For this review, take the finished solid that the model builds, in its own axes (mm). Round coordinates to 2 decimals unless told otherwise and drop trailing zeros. Write each loop counter-clockwise with the first axis right and the second up, starting at its lowest first coordinate (ties: lowest second). Pieces come first, ordered by that corner, then holes. Notation, with made-up numbers: (53.25, 35.5) -> (63.25, 35.5) arc R16 cw to (63.25, 52.5) -> close; hole circle Ø2 at (89, 30). An arc over 180 degrees is marked (long way). Answer in a Markdown table with one row per item.
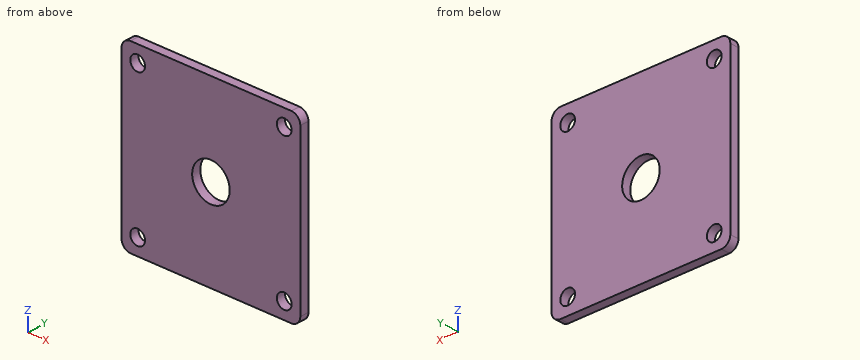
from build123d import *

# Parameters (mm, degrees)
SKETCH1_W           = 63.5
SKETCH1_H           = 63.5
BOSS_EXTRUDE1_DEPTH = 3.175
FILLET1_R           = 3.175
CUT_EXTRUDE1_REACH  = 47.013
SKETCH2_R           = 6.6675
CUT_EXTRUDE2_REACH  = 47.013
SKETCH3_R           = 2.6162


with BuildPart() as part:
    # Sketch1 → Boss-Extrude1 (new body)
    with BuildSketch(Plane(origin=(0, 0, 0), x_dir=(1, 0, 0), z_dir=(0, 1, 0))):
        Rectangle(SKETCH1_W, SKETCH1_H)
    extrude(amount=BOSS_EXTRUDE1_DEPTH)

    # Fillet1
    fillet1_edges = [part.edges().sort_by_distance(p)[0] for p in [
        (31.75, 1.5875, 31.75),
        (-31.75, 1.5875, 31.75),
        (-31.75, 1.5875, -31.75),
        (31.75, 1.5875, -31.75),
    ]]
    fillet(fillet1_edges, radius=FILLET1_R)

    # Sketch2 → Cut-Extrude1 (cut, up to next)
    with BuildSketch(Plane(origin=(0, 3.175, 0), x_dir=(1, 0, 0), z_dir=(0, 1, 0)), mode=Mode.PRIVATE) as cut_extrude1_sk1:
        with Locations(Location((0, 0, 0), (0, 0, 270))):
            Circle(SKETCH2_R)
    cut_extrude1_tool1 = extrude(cut_extrude1_sk1.sketch, amount=-CUT_EXTRUDE1_REACH, mode=Mode.PRIVATE) & part.part
    add(cut_extrude1_tool1.solids().sort_by_distance((0, 3.175, 0))[0], mode=Mode.SUBTRACT)

    # Sketch3 → Cut-Extrude2 (cut, up to next)
    with BuildSketch(Plane(origin=(0, 3.175, 0), x_dir=(1, 0, 0), z_dir=(0, 1, 0)), mode=Mode.PRIVATE) as cut_extrude2_sk1:
        with Locations(Location((26.042742751, -26.042742751, 0), (0, 0, 270))):
            Circle(SKETCH3_R)
    cut_extrude2_tool1 = extrude(cut_extrude2_sk1.sketch, amount=-CUT_EXTRUDE2_REACH, mode=Mode.PRIVATE) & part.part
    # Sketch3 → Cut-Extrude2 (cut, up to next)
    with BuildSketch(Plane(origin=(0, 3.175, 0), x_dir=(1, 0, 0), z_dir=(0, 1, 0)), mode=Mode.PRIVATE) as cut_extrude2_sk2:
        with Locations(Location((-26.042742751, -26.042742751, 0), (0, 0, 270))):
            Circle(SKETCH3_R)
    cut_extrude2_tool2 = extrude(cut_extrude2_sk2.sketch, amount=-CUT_EXTRUDE2_REACH, mode=Mode.PRIVATE) & part.part
    # Sketch3 → Cut-Extrude2 (cut, up to next)
    with BuildSketch(Plane(origin=(0, 3.175, 0), x_dir=(1, 0, 0), z_dir=(0, 1, 0)), mode=Mode.PRIVATE) as cut_extrude2_sk3:
        with Locations(Location((26.042742751, 26.042742751, 0), (0, 0, 90))):
            Circle(SKETCH3_R)
    cut_extrude2_tool3 = extrude(cut_extrude2_sk3.sketch, amount=-CUT_EXTRUDE2_REACH, mode=Mode.PRIVATE) & part.part
    # Sketch3 → Cut-Extrude2 (cut, up to next)
    with BuildSketch(Plane(origin=(0, 3.175, 0), x_dir=(1, 0, 0), z_dir=(0, 1, 0)), mode=Mode.PRIVATE) as cut_extrude2_sk4:
        with Locations(Location((-26.042742751, 26.042742751, 0), (0, 0, 90))):
            Circle(SKETCH3_R)
    cut_extrude2_tool4 = extrude(cut_extrude2_sk4.sketch, amount=-CUT_EXTRUDE2_REACH, mode=Mode.PRIVATE) & part.part
    add(cut_extrude2_tool1.solids().sort_by_distance((26.042743, 3.175, 26.042743))[0], mode=Mode.SUBTRACT)
    add(cut_extrude2_tool2.solids().sort_by_distance((-26.042743, 3.175, 26.042743))[0], mode=Mode.SUBTRACT)
    add(cut_extrude2_tool3.solids().sort_by_distance((26.042743, 3.175, -26.042743))[0], mode=Mode.SUBTRACT)
    add(cut_extrude2_tool4.solids().sort_by_distance((-26.042743, 3.175, -26.042743))[0], mode=Mode.SUBTRACT)


solid = part.part
1) Consider section C-C on y = 1.2. State how many separate pieces and enclosed holes the cut face has, then the cut area to 3 significant figures.
Solved:
| item | result |
|---|---|
| separate pieces | 1 |
| enclosed holes | 5 |
| area | 3,800 mm² |
2) For line 1 (Z direction, x = 28, y = 2.3); line 2 (Z direction, x = -27.5, y = 0.5); line 3 (X direction, y = 0.45, z = -25), list the stretches that pass through material, from the lowest coordinate up. Write a range as [from, to].
Solved:
| item | result |
|---|---|
| line 1 | [-31.75, -27.78], [-24.31, 24.31], [27.78, 31.75] |
| line 2 | [-31.75, -28.22], [-23.87, 23.87], [28.22, 31.75] |
| line 3 | [-31.75, -28.44], [-23.64, 23.64], [28.44, 31.75] |
3) Consider section D-D on z = 26. State the section outline as (x, y) points (3 decimals), then the cut area to 3 significant figures.
Solved:
| item | result |
|---|---|
| outline | (-31.75, 0) -> (-28.659, 0) -> (-28.659, 3.175) -> (-31.75, 3.175) -> close; (-23.427, 0) -> (23.427, 0) -> (23.427, 3.175) -> (-23.427, 3.175) -> close; (28.659, 0) -> (31.75, 0) -> (31.75, 3.175) -> (28.659, 3.175) -> close |
| area | 168 mm² |
